Autodesk Inventor part; units mm, degrees
ref_plane "YZ Plane" through (0, 0, 0) normal (1, 0, 0) x (0, 1, 0)
ref_plane "XZ Plane" through (0, 0, 0) normal (0, 1, 0) x (-1, 0, 0)
ref_plane "XY Plane" through (0, 0, 0) normal (0, 0, 1) x (1, 0, 0)
sketch "Sketch1" plane through (0, 0, 0) normal (0, 1, 0) x (-1, 0, 0)
  circle A0 centre (0, 0) radius 8.5
  circle A1 centre (0, 0) radius 3.5
  circle A2 centre (0, 0) radius 7
  line L0 (5.4772, 6.5) -> (1.8028, 3)
  line L1 (1.8028, -3) -> (5.4772, -6.5)
  line L2 (-1.299, 3.25) -> (-2.0392, 6.6964)
  line L3 (-2.8723, 2) -> (-6.0622, 3.5)
  line L4 (-2.8723, -2) -> (-6.0622, -3.5)
  line L5 (-1.299, -3.25) -> (-2.0392, -6.6964)
  dimension "d0" = 17
  dimension "d2" = 6
  dimension "d3" = 14
  dimension "d4" = 13
  dimension "d5" = 4
  dimension "d6" = 7
  dimension "d8" = 7
  dimension "d9" = 6.5
extrude "Extrusion1" add sketch "Sketch1" along normal blind 0.9 contours L0 A2 L1 A0 | L0 A1 L2 A2 | A2 L5 A1 L1 | L3 A1 L4 A2 picked at (-7.9468, 0.2439)
properties part number "7mm E-Clip"
Geometry check sheet. Reference: the model listing, model coordinates, mm. Give positions to 0.01 mm unless a question says otherwise; leave off trailing zeros. Order: outer loops, then holes, each group sorted by start corner. A loop starts at its lowest first (then second) coordinate and runs counter-clockwise, first axis right, second up. Notation, with made-up numbers: (-28.75, 52) -> (7.25, 52) arc R13 ccw to (7.25, 59) -> close; hole circle Ø10 at (-37, 11). An arc over 180 degrees is marked (long way). Write each question's results on one line, items separated by ' | '. Start each with the question number.
(1) Sectioned sample at A-A (x = 0). Enter the section's corners in (y, z).
(2) Sectioned sample at D-D (z = 0). Enter the section's corners in (x, y).
(3) Scan lines: line 1 (Z direction, x = 5.5, y = 0.3); line 2 (Z direction, x = 4.5, y = 0.8); line 3 (X direction, y = 0.2, z = -5). Record each from-to range of solid material in increasing order.
(4) Sectioned sample at B-B (z = -6). Enter the section's corners in (x, y), plus the area to 3 significant figures.
(5) Mould release check, pull along X, two halves, no side actions. Record for faces 1 (the face through (3.5, 0.4, 0)), 2 (the face through (8.496, 0.444, -0.27)), 3 (the face through (4.33, 0.44, -5.5)): pulls with the +X half, pulls with the -X half, needs draft (parallel to the pull), parting line crosses it, or undercut.
(6) Gauge pin test, flat end, axial feed: P1, Ø1, axis at x = 2.5, z = 1.5, coming from the +Y side. Record the tip position at first contact, or that the pin passes through.
(7) Sectioned sample at C-C (x = 3.75). Enter the section's corners in (y, z), plus the area to 3 significant figures.
Answer below:
1) outline: (0, -8.5) -> (0.9, -8.5) -> (0.9, -3.5) -> (0, -3.5) -> close; (0, 3.5) -> (0.9, 3.5) -> (0.9, 8.5) -> (0, 8.5) -> close
2) outline: (3.5, 0) -> (8.5, 0) -> (8.5, 0.9) -> (3.5, 0.9) -> close
3) line 1: -6.48 to -4.33, -3.24 to 3.24, 4.33 to 6.48 | line 2: -7.21 to -5.36, -2.77 to 2.77, 5.36 to 7.21 | line 3: -3.9 to 1.67, 4.9 to 6.87
4) outline: (-4.95, 0) -> (1.89, 0) -> (1.89, 0.9) -> (-4.95, 0.9) -> close; (3.61, 0) -> (6.02, 0) -> (6.02, 0.9) -> (3.61, 0.9) -> close | area: 8.33 mm2
5) face 1: pulls with the -X half | face 2: parting line crosses it | face 3: undercut
6) P1: through
7) outline: (0, -7.63) -> (0.9, -7.63) -> (0.9, -5.91) -> (0, -5.91) -> close; (0, -2.41) -> (0.9, -2.41) -> (0.9, 2.41) -> (0, 2.41) -> close; (0, 5.91) -> (0.9, 5.91) -> (0.9, 7.63) -> (0, 7.63) -> close | area: 7.43 mm2
